Geometry check sheet. Reference: drawing and pictorial views, mm from the part's lowest x, y, z. Give positions to 0.01 mm unless a question says otherwise; leave off trailing zeros. Order: outer loops, then holes, each group sorted by start corner. A loop starts at its lowest first (then second) coordinate and runs counter-clockwise, first axis right, second up. Notation, with made-up numbers: (44, 37.25) -> (48, 37.25) arc R32 cw to (48, 67.25) -> close; hole circle Ø5 at (52, 78). An arc over 180 degrees is marked (long way). Write each question's results on one line, items separated by ' | '.
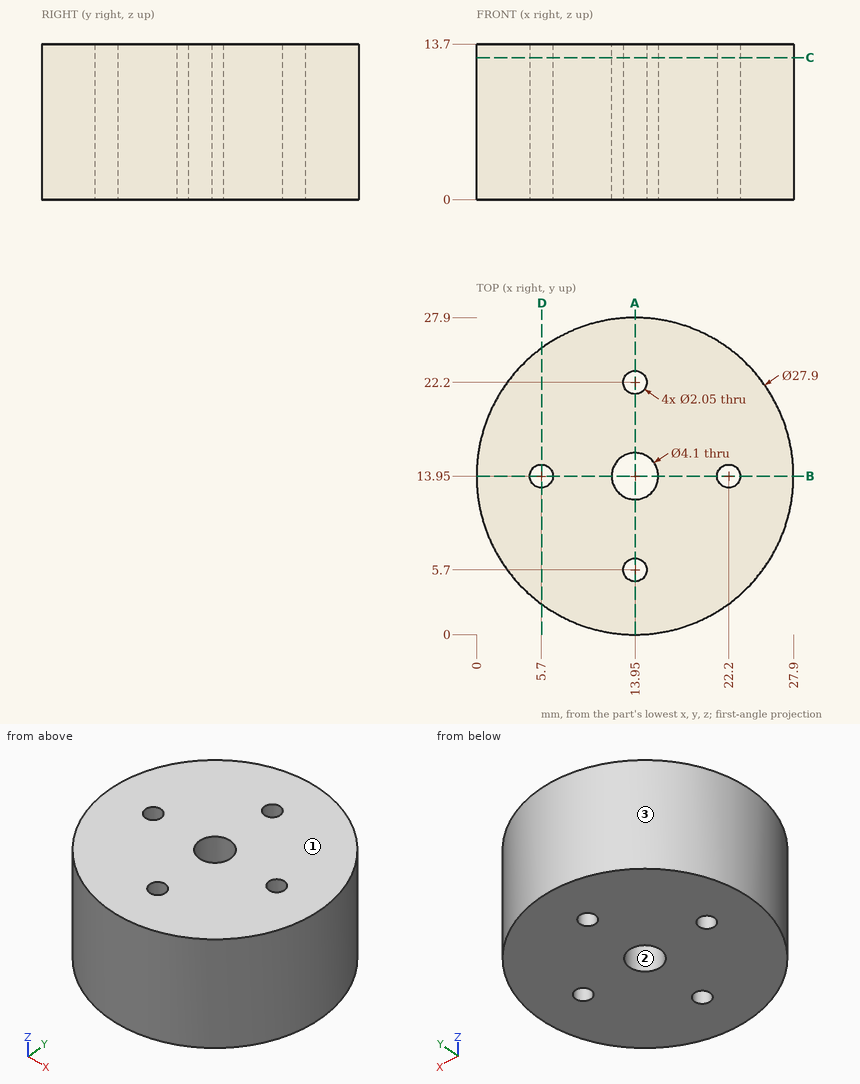
1. Section check D-D on x = 5.75. Record the cut outline in (y, z), then the cut area to 3 significant figures.
Verdict:
outline: (2.66, 0) -> (12.93, 0) -> (12.93, 13.7) -> (2.66, 13.7) -> close; (14.97, 0) -> (25.24, 0) -> (25.24, 13.7) -> (14.97, 13.7) -> close | area: 281 mm^2
2. Section check C-C on z = 12.5. Record the cut outline in (x, y) (3 decimals), then the cut area to 3 significant figures.
Verdict:
outline: circle Ø27.9 at (13.95, 13.95); hole circle Ø2.05 at (5.7, 13.95); hole circle Ø4.1 at (13.95, 13.95); hole circle Ø2.05 at (13.95, 5.7); hole circle Ø2.05 at (13.95, 22.2); hole circle Ø2.05 at (22.2, 13.95) | area: 585 mm^2
3. Material ranges on probe 1 along Y at (x, z) = (13.95, 4.75) (3 decimals); probe 2 along X at (y, z) = (23, 13.25); probe 3 along X at (y, z) = (15.75, 4.25), recorded low to high. Write a range as from..to.
Verdict:
probe 1: y = 0..4.675, 6.725..11.9, 16..21.175, 23.225..27.9 | probe 2: x = 3.33..13.31, 14.59..24.57 | probe 3: x = 0.12..12.97, 14.93..27.78
4. Section check A-A on x = 13.95. Record the cut outline in (y, z) (3 decimals).
Verdict:
outline: (0, 0) -> (4.675, 0) -> (4.675, 13.7) -> (0, 13.7) -> close; (6.725, 0) -> (11.9, 0) -> (11.9, 13.7) -> (6.725, 13.7) -> close; (16, 0) -> (21.175, 0) -> (21.175, 13.7) -> (16, 13.7) -> close; (23.225, 0) -> (27.9, 0) -> (27.9, 13.7) -> (23.225, 13.7) -> close
5. Gauge pin test, flat ends, axial feed: pin 1 Ø1 at (y, z) = (22, 10.5) entering from +X; pin 2 Ø4 at (x, z) = (22.5, 9.5) entering from -Y; pin 3 Ø5 at (y, z) = (24.5, 6) entering from -X. Record the tip position at first contact, or that the pin passes through.
Verdict:
pin 1: stops at x = 25.68 | pin 2: stops at y = 1.63 | pin 3: stops at x = 2.56
6. Mould release check, pull along Y, two halves, no side actions. Record for the marked faces 1, 2 and 3: +Y half, -Y half, draft (parallel to the pull), parting line (faces both ways), or undercut.
Verdict:
face 1: draft | face 2: undercut | face 3: parting line
